Check sheet for the modelled part. Datum: model origin and axes. Units: mm. A direction names the side the tool comes from. Give positions to 0.01 mm unless a question says otherwise; leave off trailing zeros. Write each loop counter-clockwise with the first axis right and the second up, starting at its lowest first coordinate (ties: lowest second). Pieces come first, ordered by that corner, then holes. Notation, with made-up numbers: M -16.75,56 L 13.25,56 A27 cw 13.25,86 Z; hole C 48.25,37 d10. An arc over 180 degrees is marked long. One line per item, written item: value. Start each with the question number.
Autodesk Inventor part; units mm, degrees
ref_plane "YZ Plane" through (0, 0, 0) normal (1, 0, 0) x (0, 1, 0)
ref_plane "XZ Plane" through (0, 0, 0) normal (0, 1, 0) x (-1, 0, 0)
ref_plane "XY Plane" through (0, 0, 0) normal (0, 0, 1) x (1, 0, 0)
sketch "Sketch2" plane through (0, 0, 0) normal (0, 0, 1) x (1, 0, 0)
  line L0 (0, 278.716) -> (197.082, 197.082) construction
  line L1 (197.082, 197.082) -> (278.716, 0) construction
  line L2 (278.716, 0) -> (197.082, -197.082) construction
  line L3 (197.082, -197.082) -> (0, -278.716) construction
  line L4 (0, -278.716) -> (-197.082, -197.082) construction
  line L5 (-197.082, -197.082) -> (-278.716, 0) construction
  line L6 (-278.716, 0) -> (-197.082, 197.082) construction
  line L7 (-197.082, 197.082) -> (0, 278.716) construction
  line L8 (-197.082, 197.082) -> (0, 278.716) construction
  line L9 (-461.6493, 774.8136) -> (-221.4406, 874.3113) construction
  line L10 (-98.541, 237.899) -> (-341.545, 824.5625) construction
  line L11 (-221.4406, 874.3113) -> (0, 874.3113) construction
  line L12 (0, 874.3113) -> (0, 278.716) construction
  line L13 (-461.6493, 774.8136) -> (-618.2315, 618.2315) construction
  line L14 (-618.2315, 618.2315) -> (-197.082, 197.082) construction
  line L15 (-223.3864, 868.0934) -> (-339.6315, 819.9431)
  line L16 (-5, 869.3113) -> (-217.2635, 869.3113)
  line L17 (-455.8767, 771.7928) -> (-339.6315, 819.9431)
  line L18 (-611.1604, 618.2315) -> (-461.0675, 768.3244)
  arc A0 (-217.2635, 869.3113) -> (-223.3864, 868.0934) centre (-217.2635, 853.3113) ccw
  arc A1 (-455.8767, 771.7928) -> (-461.0675, 768.3244) centre (-449.7538, 757.0107) ccw
  point P0 (0, 0)
  point P1 (0, 0)
  point P2 (0, 0)
  point P3 (-220.4461, 869.3113)
  point P4 (-458.817, 770.5748)
  dimension "d0" = 515
  dimension "d1" = 260
  dimension "d2" = 635
  dimension "d6" = 5
  dimension "d10" = 5
  dimension "d14" = 5
  dimension "d15" = 16
contour flange "Contour Flange1" sketch "Sketch2" thickness 8 bend radius 8 width 80 along (0, 0, 1) mid plane no both sides no wall seen from (-111.1317, 869.3113, 0) lies toward (0, -1, 0) curves L16 A0 L15 L17 A1 L18
bend "Bend1"
corner "Corner1"
sketch "Sketch3" plane through (-455.8767, 771.7928, 80) normal (-0.3826834, 0.9238795, 0) x (0.9238795, 0.3826834, 0)
  line L0 (125.8228, 80) -> (125.8228, 0) construction
  line L1 (0, 0) -> (251.6457, 0)
  circle A0 centre (43.3228, 40) radius 10
  circle A1 centre (208.3228, 40) radius 10
  point P0 (125.8228, 40)
  dimension "d27" = 20
  dimension "d28" = 82.5
extrude "Extrusion1" [suppressed]
equation "\"d0\" = Барабан_размер_по_плоскостям"
equation "\"d1\" = Кассета_длина_грани"
equation "\"d2\" = Кассета_высота"
equation "\"d10\" = d6"
equation "\"d15\" = BendRadius + Thickness"
equation "\"d16\" = Thickness"
equation "\"d17\" = BendReliefWidth"
equation "\"d18\" = BendReliefDepth"
equation "\"d19\" = MinimumRemnant"
equation "\"d20\" = TransitionRadius"
equation "\"d22\" = BendRadius"
equation "\"d24\" = CornerReliefSize"
equation "\"d25\" = GapSize"
equation "\"d26\" = JacobiRadiusSize"
equation "\"BendRadius\" = Thickness"
equation "\"BendReliefWidth\" = Thickness"
equation "\"BendReliefDepth\" = 0.5 * Thickness"
equation "\"CornerReliefSize\" = 4 * Thickness"
equation "\"MinimumRemnant\" = 2 * Thickness"
equation "\"TransitionRadius\" = BendRadius"
equation "\"JacobiRadiusSize\" = BendRadius"
equation "\"GapSize\" = Thickness"
properties part number "DMF 01 52 Top sheet v2.1"
1) Cross-section at C-C (y = 800.5). Record the boundary of the cut face in (x, z).
2) Cross-section at A-A (z = 32). Record the boundary of the cut face in (x, y).
3) Cross-section at B-B (x = -51.5). Record the boundary of the cut face in (y, z), plus the area to 3 significant figures.
4) Gauge pin test, flat ends, axial feed: pin 1 (6 mm diameter, centred on x = -250, z = 44, fed in from -Y); pin 2 (5 mm diameter, centred on y = 748, z = 34, fed in from -X); pin 3 (4 mm diameter, centred on x = -532.5, z = 65, fed in from +Y). Record the tip position at first contact, or that the pin passes through.
5) Material ranges on L1, parallel to Y at x = -197, z = 32; L2, parallel to Y at x = -229, z = 8.5; L3, parallel to X at y = 734.5, z = 36, recorded low to high. Write a range as from..to.
6) Tool access check on faces 1 (the flat face through (-110, 861.311, 39)), 2 (the flat face through (-110, 869.311, 39)). Record the directions out of +Z, -Z, +X, -X, +Y, -Y that give a thin tool (end or side, any length) a straight path to the whole face; none if there is none.
Data:
1. outline: M -386.57,0 L -365.67,0 L -365.67,80 L -386.57,80 Z
2. outline: M -611.16,618.23 L -605.5,612.57 L -455.41,762.67 A8 cw -452.82,764.4 L -336.57,812.55 L -220.33,860.7 A8 cw -217.26,861.31 L -5,861.31 L -5,869.31 L -217.26,869.31 A16 ccw -223.39,868.09 L -339.63,819.94 L -455.88,771.79 A16 ccw -461.07,768.32 Z
3. outline: M 861.31,0 L 869.31,0 L 869.31,80 L 861.31,80 Z
3. area: 640 mm2
4. pin 1: stops at y = 847.17
4. pin 2: stops at x = -483.89
4. pin 3: stops at y = 698.89
5. L1: y = 861.31..869.31
5. L2: y = 857.11..865.77
5. L3: x = -494.89..-483.58
6. face 1: +Z, -Z, +X, -Y
6. face 2: +Z, -Z, +X, -X, +Y
